Autodesk Inventor part; units mm, degrees
ref_plane "YZ Plane" through (0, 0, 0) normal (1, 0, 0) x (0, 1, 0)
ref_plane "XZ Plane" through (0, 0, 0) normal (0, 1, 0) x (-1, 0, 0)
ref_plane "XY Plane" through (0, 0, 0) normal (0, 0, 1) x (1, 0, 0)
sketch "Skizze4" plane through (0, 0, 0) normal (0, 0, 1) x (1, 0, 0)
  line L0 (2.5046, -1.4353) -> (0.0093, -2.8867)
  line L1 (0.0093, -2.8867) -> (-2.4953, -1.4514)
  line L2 (-2.4953, -1.4514) -> (-2.5046, 1.4353)
  line L3 (-2.5046, 1.4353) -> (-0.0093, 2.8867)
  line L4 (-0.0093, 2.8867) -> (2.4953, 1.4514)
  line L5 (2.4953, 1.4514) -> (2.5046, -1.4353)
  point P0 (0, 0)
  point P1 (0, 0)
  dimension "d21" = 5
extrude "Extrusion1" add sketch "Skizze4" along normal blind 1
sketch "Skizze5" plane through (0, 0, 0) normal (0, 0, -1) x (-1, 0, 0)
  circle A0 centre (0, 0) radius 2
  dimension "d7" = 4
extrude "Extrusion2" add sketch "Skizze5" along normal blind 5.5
sketch "Skizze6" plane through (0, 0, 1) normal (0, 0, 1) x (1, 0, 0)
  point P0 (0, 0)
hole "Bohrung1" at (0, 0, 1) direction (0, 0, -1) diameter 3.4 depth 10.65 tip angle 118
thread "Gewinde2"
properties part number "huelse_M3"
Verification items for the finished model (mm, model axes). A direction names the side the tool comes from. Coordinates: 2 decimals unless noted, no trailing zeros. Order: outer loops, then holes, each group sorted by start corner. A loop starts at its lowest first (then second) coordinate and runs counter-clockwise, first axis right, second up. Notation, with made-up numbers: (51, 14.25) -> (72, 14.25) arc R18 cw to (72, 49.25) -> close; hole circle Ø9 at (-17, -24.75). An arc over 180 degrees is marked (long way). Use CSV: the item, a comma, the result in double quotes. Start each with the question number.
Q1. Section check B-B, the plane z = -0.75. Record the cut outline in (x, y).
Q2. Section check A-A, the plane y = 1.6. Record the cut outline in (x, z), and give its area (3 significant figures).
Q3. Section check C-C, the plane y = 0.8. Record the cut outline in (x, z), and give its area (3 significant figures).
Q4. Tool access check on faces 5 (the flat face through (-2, 0, 1)), 6 (the flat face through (-1, -2, 0)). Record the directions out of +Z, -Z, +X, -X, +Y, -Y that give a thin tool (end or side, any length) a straight path to the whole face; none if there is none.
Q5. Draft check along X on faces 1 (the flat face through (1.225, 2.179, 0.493)), 2 (the cylindrical face through (0, 2, -3)), 3 (the flat face through (-1.225, -2.179, 0.493)), 4 (the cylindrical face through (1.66, 0.37, -2.3)). Enter one of: +X half, -X half, draft (parallel to the pull), parting line (faces both ways), or undercut.
Q6. Depth check by flat-ended pin: P1, Ø3, axis at y = -2, z = -4.5, coming from the +X side; P2, Ø1.5, axis at x = -0.5, y = 0, coming from the -Z side; P3, Ø2, axis at y = 2, z = -3, coming from the -X side. Enter the tip coordinate at first touch or a pass-through.
Q7. Section check D-D, the plane y = -1.85. Record the cut outline in (x, z), and give its area (3 significant figures).
Q8. Thickness scan on line 1 along Y through (x, z) = (0, -2); line 2 along Z through (x, y) = (-2, 1.65); line 3 along Y through (x, z) = (1.2, 0.75). Record the ranges inside material, lowest first.
Returned:
1,outline,"circle Ø4 at (0, 0); hole circle Ø3.4 at (0, 0)"
2,outline,"(-2.22, 0) -> (-1.2, 0) -> (-1.2, -5.5) -> (-0.57, -5.5) -> (-0.57, 1) -> (-2.22, 1) -> close; (0.57, -5.5) -> (1.2, -5.5) -> (1.2, 0) -> (2.24, 0) -> (2.24, 1) -> (0.57, 1) -> close"
2,area,"10.2 mm^2"
3,outline,"(-2.5, 0) -> (-1.83, 0) -> (-1.83, -5.5) -> (-1.5, -5.5) -> (-1.5, 1) -> (-2.5, 1) -> close; (1.5, -5.5) -> (1.83, -5.5) -> (1.83, 0) -> (2.5, 0) -> (2.5, 1) -> (1.5, 1) -> close"
3,area,"5.66 mm^2"
4,face 5,"+Z, +X, -X, +Y, -Y"
4,face 6,"-Z"
5,face 1,"+X half"
5,face 2,"parting line"
5,face 3,"-X half"
5,face 4,"undercut"
6,P1,"stops at x = 1.94"
6,P2,"passes through"
6,P3,"stops at x = -1.73"
7,outline,"(-1.8, 0) -> (-0.76, 0) -> (-0.76, -5.5) -> (0.76, -5.5) -> (0.76, 0) -> (1.79, 0) -> (1.79, 1) -> (-1.8, 1) -> close"
7,area,"12.0 mm^2"
8,line 1,"y = -2 to -1.7, 1.7 to 2"
8,line 2,"z = 0 to 1"
8,line 3,"y = -2.19 to -1.2, 1.2 to 2.19"
